```python
from build123d import *

# Parameters (mm, degrees)
F1_DEPTH      = 12.5
F1_DEPTH_BACK = 12.5


with BuildPart() as f1:
    # F0 (on Right) → F1 (new body, two sides)
    with BuildSketch(Plane.YZ) as f1_sk:
        with BuildLine():
            ThreePointArc((9.632908, 11.806406), (9.732809, 11.047587), (9.266883, 10.440381))
            Line((9.266883, 10.440381), (-8.053625, 0.440381))
            ThreePointArc((-8.053625, 0.440381), (-8.812444, 0.34048), (-9.41965, 0.806406))
            Line((-9.41965, 0.806406), (-10.454072, 2.598076))
            ThreePointArc((-10.454072, 2.598076), (-12.140511, 3.297186), (-13.253109, 1.849789))
            Line((-13.253109, 1.849789), (-13.256593, -1.202352))
            ThreePointArc((-13.256593, -1.202352), (-12.671615, -2.618041), (-11.256594, -3.204635))
            Line((-11.256594, -3.204635), (11.598487, -3.204635))
            ThreePointArc((11.598487, -3.204635), (13.012701, -2.618849), (13.598487, -1.204635))
            Line((13.598487, -1.204635), (13.598487, 10.531089))
            ThreePointArc((13.598487, 10.531089), (12.573361, 13.005963), (10.098487, 14.031089))
            Line((10.098487, 14.031089), (10.080538, 14.031089))
            ThreePointArc((10.080538, 14.031089), (9.214513, 13.531089), (9.214513, 12.531089))
            Line((9.214513, 12.531089), (9.632908, 11.806406))
        make_face()
        with BuildLine():
            Line((10.098487, 7.745081), (10.098487, 0.795365))
            ThreePointArc((10.098487, 0.795365), (9.512701, -0.618849), (8.098487, -1.204635))
            Line((8.098487, -1.204635), (-4.999951, -1.204635))
            ThreePointArc((-4.999951, -1.204635), (-5.482408, -0.835916), (-5.253301, -0.273574))
            Line((-5.253301, -0.273574), (-3.200361, 0.933013))
            Line((-3.200361, 0.933013), (-1.584336, 1.866025))
            Line((-1.584336, 1.866025), (9.348487, 8.178094))
            ThreePointArc((9.348487, 8.178094), (9.848487, 8.178094), (10.098487, 7.745081))
        make_face(mode=Mode.SUBTRACT)
    extrude(amount=F1_DEPTH)
    extrude(f1_sk.sketch, amount=-F1_DEPTH_BACK)


solid = f1.part
```
For this review, take the finished solid that the model builds, in its own axes (mm). A direction names the side the tool comes from. Coordinates: 2 decimals unless noted, no trailing zeros. Loops run counter-clockwise (first coordinate to the right, second up) from the corner with the lowest first, then second, coordinate; pieces in that order, holes last. Notation, with made-up numbers: (-10.75, -36) - (1.25, -36) arc R34 cw to (1.25, -4) - close; hole circle Ø7 at (-30.75, -39). An arc over 180 degrees is marked (long way). Use one line per item in the form item = value. Start each with the question number.
1) Take a section at D-D (z = 3). State the section outline as (x, y) points, plus the area to 3 significant figures.
2) For faces 1 (the face through (0.175, 9.736, 11.058)), 2 (the face through (0.18, -4.24, 0.32)), 3 (the face through (0.18, -9.93, 1.69)), list the 3-axis set-ups (+Z, -Z, +X, -X, +Y, -Y) from which the entire face can be reached by the end or side of a thin tool; tool diameter is ignored.
3) To check wall thickness, follow probe 1 along Y at (x, z) = (-3.5, 0.5); probe 2 along Y at (x, z) = (6, 6); probe 3 along Z at (x, y) = (-7.75, 6.75). State the ranges of each line that lie inside material, in increasing order. Write a range as from..to.
4) Take a section at B-B (y = -2.75). State the section outline as (x, z) points.
5) Draft analysis for pull direction Y (two halves, no side actions). For faces 4 (the face through (-12.5, 1, 4)), 5 (the face through (0.18, 12.6, 12.98)), 6 (the face through (0, 10.098, 4)), state which applies: released by +Y, released by -Y, zero draft, split by the parting line, or undercut.
6) For pin 1 (10 mm diameter, centred on y = 4.5, z = 8, fed in from -X); pin 2 (1.5 mm diameter, centred on x = -7.5, y = -0.5, fed in from +Z); pin 3 (3.5 mm diameter, centred on x = 0, z = 5.5, fed in from -Y), all flat-tipped, find the tip position at first contact; note any pin that passes through.
7) Take a section at C-C (z = 6). State the section outline as (x, y) points.
From the geometry:
q1.outline = (-12.5, -12.71) - (12.5, -12.71) - (12.5, -10.79) - (-12.5, -10.79) - close; (-12.5, -3.62) - (12.5, -3.62) - (12.5, 0.38) - (-12.5, 0.38) - close; (-12.5, 10.1) - (12.5, 10.1) - (12.5, 13.6) - (-12.5, 13.6) - close
q1.area = 236 mm2
q2.face_1 = +X, -X, -Y
q2.face_2 = +X, -X
q2.face_3 = +Z, +X, -X
q3.probe_1 = -13.25..-9.14, -7.95..-3.94, 10.08..13.6
q3.probe_2 = 1.58..5.58, 10.1..13.6
q3.probe_3 = -3.2..-1.2, 6.68..8.99
q4.outline = (-12.5, -3.2) - (12.5, -3.2) - (12.5, -1.2) - (-12.5, -1.2) - close; (-12.5, 1.19) - (12.5, 1.19) - (12.5, 3.5) - (-12.5, 3.5) - close
q5.face_4 = zero draft
q5.face_5 = released by +Y
q5.face_6 = undercut
q6.pin_1 = -12.5
q6.pin_2 = 5.23
q6.pin_3 = -2.32
q7.outline = (-12.5, 1.58) - (12.5, 1.58) - (12.5, 5.58) - (-12.5, 5.58) - close; (-12.5, 10.1) - (12.5, 10.1) - (12.5, 13.6) - (-12.5, 13.6) - close
